CAD build for the part. Positions are in the model's coordinates, mm. A direction names the side the tool comes from. Round coordinates to 2 decimals unless told otherwise and drop trailing zeros. Write each loop counter-clockwise with the first axis right and the second up, starting at its lowest first coordinate (ties: lowest second). Pieces come first, ordered by that corner, then holes. Notation, with made-up numbers: (24, 17) - (37, 17) arc R19 cw to (37, 37) - close; hole circle Ø8 at (67, 62). An arc over 180 degrees is marked (long way). Put each result on its own line as item: value. Start each with the question number.
Item 1: Cut at A-A (x = 0). Give the cut face in (y, z).
Item 2: Mould opens along Z. For faces 3 (the cylindrical face through (-9.76, 121.62, -2.17)), 4 (the flat face through (0, 50, 9)), 5 (the flat face through (0, 60, 0)), 6 (the cylindrical face through (0.33, 24.65, -7.493)) say: released by +Z, released by -Z, zero draft, split by the parting line, or undercut.
Item 3: Cut at D-D (y = 19.5). Give the cut face in (x, z), and give its area (3 significant figures).
Item 4: Drill centre lines: line 1 (X direction, y = 91, z = 0); line 2 (Y direction, x = 9.5, z = 4); line 3 (Y direction, x = -12.5, z = -11.5). Where is each one in solid material? Low to high. Write a range as from..to.
Item 5: Cut at C-C (y = 153). Give the cut face in (x, z), and give its area (3 significant figures).
Item 6: Pin check, flat tips, straight feed: pin 1 Ø1 at (x, y) = (6.5, 152.5) entering from -Z; pin 2 Ø12 at (y, z) = (34.5, 5) entering from -X; pin 3 Ø2 at (x, y) = (-5.5, 128) entering from +Z; pin 4 Ø2 at (y, z) = (111, -14) entering from +X. Stop position of each tip, or through.
Item 7: 3-axis set-ups, long thin cutter, end or side, ignore diameter. For faces 1 (the cylindrical face through (3.604, 121.625, 11.446)), 2 (the flat face through (9, 185, -5)): which of +Z, -Z, +X, -X, +Y, -Y reach the whole face in a straight line?
Item 8: Cut at B-B (z = 0). Give the cut face in (x, y), and give its area (3 significant figures).
```python
from build123d import *

# Parameters (mm, degrees)
SKETCH1_R           = 7.5
BOSS_EXTRUDE1_DEPTH = 50
SKETCH2_R           = 21.183921509
BOSS_EXTRUDE2_DEPTH = 10
SKETCH3_R           = 12
SKETCH3_R_2         = 10
BOSS_EXTRUDE3_DEPTH = 125


with BuildPart() as part:
    # Sketch1 → Boss-Extrude1 (new body)
    with BuildSketch(Plane(origin=(0, 0, 0), x_dir=(1, 0, 0), z_dir=(0, 1, 0))):
        with Locations(Location((0, 0, 0), (0, 0, 270))):
            Circle(SKETCH1_R)
    extrude(amount=BOSS_EXTRUDE1_DEPTH)

    # Sketch2 → Boss-Extrude2 (add)
    with BuildSketch(Plane(origin=(0, 50, 0), x_dir=(1, 0, 0), z_dir=(0, 1, 0))):
        with Locations(Location((0, 0, 0), (0, 0, 270))):
            Circle(SKETCH2_R)
    extrude(amount=BOSS_EXTRUDE2_DEPTH)

    # Sketch3 → Boss-Extrude3 (add)
    with BuildSketch(Plane(origin=(0, 60, 0), x_dir=(1, 0, 0), z_dir=(0, 1, 0))):
        with Locations(Location((0, 0, 0), (0, 0, 270))):
            Circle(SKETCH3_R)
        with Locations(Location((0, 0, 0), (0, 0, 270))):
            Circle(SKETCH3_R_2, mode=Mode.SUBTRACT)
    extrude(amount=BOSS_EXTRUDE3_DEPTH)


solid = part.part
```
Output values:
1. outline: (0, -7.5) - (50, -7.5) - (50, -21.18) - (60, -21.18) - (60, -12) - (185, -12) - (185, -10) - (60, -10) - (60, 10) - (185, 10) - (185, 12) - (60, 12) - (60, 21.18) - (50, 21.18) - (50, 7.5) - (0, 7.5) - close
2. face 3: undercut
2. face 4: zero draft
2. face 5: undercut
2. face 6: split by the parting line
3. outline: circle Ø15 at (0, 0)
3. area: 177 mm2
4. line 1: -12..-10, 10..12
4. line 2: 50..185
4. line 3: 50..60
5. outline: circle Ø24 at (0, 0); hole circle Ø20 at (0, 0)
5. area: 138 mm2
6. pin 1: z = -10.39
6. pin 2: x = -7.5
6. pin 3: z = 11.12
6. pin 4: through
7. face 1: +Y
7. face 2: +Z, -Z, +X, -X, +Y
8. outline: (-21.18, 50) - (-7.5, 50) - (-7.5, 0) - (7.5, 0) - (7.5, 50) - (21.18, 50) - (21.18, 60) - (12, 60) - (12, 185) - (10, 185) - (10, 60) - (-10, 60) - (-10, 185) - (-12, 185) - (-12, 60) - (-21.18, 60) - close
8. area: 1,670 mm2
